Source: CAD feature listing. Evaluate the final solid. Frame: model axes, mm. Round coordinates to 2 decimals unless told otherwise and drop trailing zeros. Order: outer loops, then holes, each group sorted by start corner. A loop starts at its lowest first (then second) coordinate and runs counter-clockwise, first axis right, second up. Notation, with made-up numbers: (61, 60) -> (120, 60) arc R25 ccw to (120, 78) -> close; hole circle Ø7 at (-13, -9.75). An arc over 180 degrees is marked (long way). Write item = value, one per line. Start each with the question number.
(1) Contact query for a flat-ended pin moving along its axis: pin 1 Ø3 at (x, z) = (15, 2) entering from +Y. Output: stop coordinate, or through.
(2) Cut plane A-A on x = 103. Return the cut outline in (y, z).
(3) Ray query, line 1 (X direction, y = 38, z = 0.3); line 2 (Y direction, x = -55.5, z = 4.3); line 3 (X direction, y = 19, z = 3.05). Return the intervals inside material, ascending.
(4) Cut plane C-C on x = -185. Return the cut outline in (y, z), then the cut area to 3 significant figures.
(5) Cut plane B-B on y = 29.5. Return the cut outline in (x, z), then the cut area to 3 significant figures.
(6) Cut plane D-D on z = 4.25. Give the number of separate pieces and of enclosed holes in the cut face, then the cut area to 3 significant figures.
from build123d import *

# Parameters (mm, degrees)
EXTRUDE_1_DEPTH = 6
FILLET_1_R      = 5


with BuildPart() as part:
    # 草图1 → 凸台-拉伸1 (new body)
    with BuildSketch(Plane.XY):
        Polygon((-170, 15), (170, 15), (170, 65), (200, 65), (200, -15), (-200, -15), (-200, 65), (-170, 65), align=None)
        with BuildLine():
            Line((-35, 7.5), (35, 7.5))
            ThreePointArc((35, 7.5), (42.5, 0), (35, -7.5))
            Line((35, -7.5), (-35, -7.5))
            ThreePointArc((-35, -7.5), (-42.5, 0), (-35, 7.5))
        make_face(mode=Mode.SUBTRACT)
        with BuildLine():
            Line((55, 7.5), (165, 7.5))
            ThreePointArc((165, 7.5), (172.5, 0), (165, -7.5))
            Line((165, -7.5), (55, -7.5))
            ThreePointArc((55, -7.5), (47.5, 0), (55, 7.5))
        make_face(mode=Mode.SUBTRACT)
        with BuildLine():
            Line((189.5, 50), (189.5, 0))
            ThreePointArc((189.5, 0), (185, -4.5), (180.5, 0))
            Line((180.5, 0), (180.5, 50))
            ThreePointArc((180.5, 50), (185, 54.5), (189.5, 50))
        make_face(mode=Mode.SUBTRACT)
        with BuildLine():
            Line((-189.5, 50), (-189.5, 0))
            ThreePointArc((-189.5, 0), (-185, -4.5), (-180.5, 0))
            Line((-180.5, 0), (-180.5, 50))
            ThreePointArc((-180.5, 50), (-185, 54.5), (-189.5, 50))
        make_face(mode=Mode.SUBTRACT)
        with BuildLine():
            Line((-55, 7.5), (-165, 7.5))
            ThreePointArc((-165, 7.5), (-172.5, 0), (-165, -7.5))
            Line((-165, -7.5), (-55, -7.5))
            ThreePointArc((-55, -7.5), (-47.5, 0), (-55, 7.5))
        make_face(mode=Mode.SUBTRACT)
    extrude(amount=EXTRUDE_1_DEPTH)

    # 圆角1
    fillet_1_edges = [part.edges().sort_by_distance(p)[0] for p in [
        (170, 65, 3),
        (200, 65, 3),
        (200, -15, 3),
        (-200, -15, 3),
        (-200, 65, 3),
        (-170, 65, 3),
        (-170, 15, 3),
        (170, 15, 3),
    ]]
    fillet(fillet_1_edges, radius=FILLET_1_R)


solid = part.part
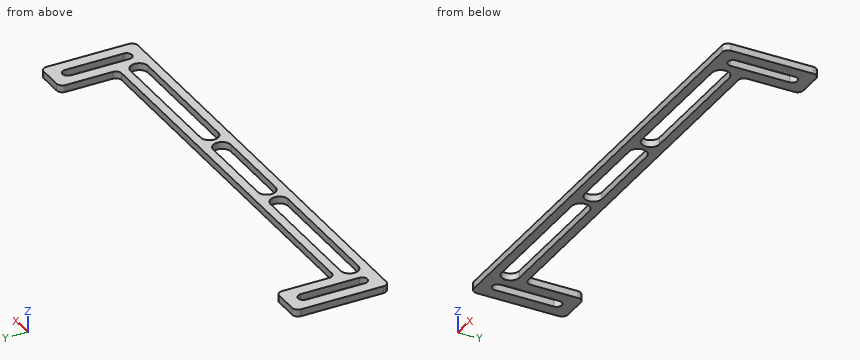
Evaluation:
q1.pin_1 = 15
q2.outline = (-15, 0) -> (-7.5, 0) -> (-7.5, 6) -> (-15, 6) -> close; (7.5, 0) -> (15, 0) -> (15, 6) -> (7.5, 6) -> close
q3.line_1 = -200 to -189.5, -180.5 to -170, 170 to 180.5, 189.5 to 200
q3.line_2 = -15 to -7.5, 7.5 to 15
q3.line_3 = -200 to -189.5, -180.5 to -169.9, 169.9 to 180.5, 189.5 to 200
q4.outline = (-15, 0) -> (-4.5, 0) -> (-4.5, 6) -> (-15, 6) -> close; (54.5, 0) -> (65, 0) -> (65, 6) -> (54.5, 6) -> close
q4.area = 126 mm^2
q5.outline = (-200, 0) -> (-189.5, 0) -> (-189.5, 6) -> (-200, 6) -> close; (-180.5, 0) -> (-170, 0) -> (-170, 6) -> (-180.5, 6) -> close; (170, 0) -> (180.5, 0) -> (180.5, 6) -> (170, 6) -> close; (189.5, 0) -> (200, 0) -> (200, 6) -> (189.5, 6) -> close
q5.area = 252 mm^2
q6.separate_pieces = 1
q6.enclosed_holes = 5
q6.area = 9,070 mm^2
